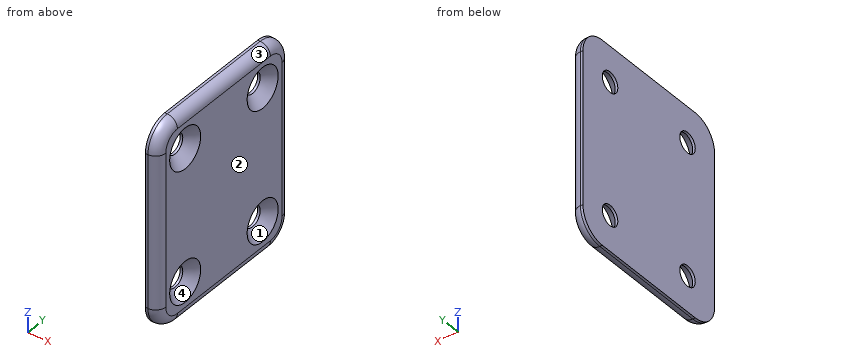
from build123d import *

# Parameters (mm, degrees)
CYLINDER005_R     = 2
CYLINDER005_DEPTH = 30
CYLINDER006_R     = 2
CYLINDER006_DEPTH = 30
CYLINDER007_R     = 2
CYLINDER007_DEPTH = 30
CYLINDER004_R     = 2
CYLINDER004_DEPTH = 30
BOX001_W          = 2.5
BOX001_H          = 34
BOX001_DEPTH      = 40
FILLET006_R       = 5
CHAMFER006_SIZE   = 2
FILLET007_R       = 2


with BuildPart() as obj1:
    # Cylinder005 → Cylinder005 (new body)
    with BuildSketch(Plane(origin=(20, -10, 6), x_dir=(0, 0, -1), z_dir=(1, 0, 0))):
        Circle(CYLINDER005_R)
    extrude(amount=CYLINDER005_DEPTH)


with BuildPart() as obj2:
    # Cylinder006 → Cylinder006 (new body)
    with BuildSketch(Plane(origin=(20, -10, 32), x_dir=(0, 0, -1), z_dir=(1, 0, 0))):
        Circle(CYLINDER006_R)
    extrude(amount=CYLINDER006_DEPTH)


with BuildPart() as obj3:
    # Cylinder007 → Cylinder007 (new body)
    with BuildSketch(Plane(origin=(20, 10, 6), x_dir=(0, 0, -1), z_dir=(1, 0, 0))):
        Circle(CYLINDER007_R)
    extrude(amount=CYLINDER007_DEPTH)


with BuildPart() as obj4:
    # Cylinder004 → Cylinder004 (new body)
    with BuildSketch(Plane(origin=(20, 10, 32), x_dir=(0, 0, -1), z_dir=(1, 0, 0))):
        Circle(CYLINDER004_R)
    extrude(amount=CYLINDER004_DEPTH)

    # Fusion003: union obj1, obj2, obj3
    add(obj1.part)
    add(obj2.part)
    add(obj3.part)


with BuildPart() as obj5:
    # Box001 → Box001 (new body)
    with BuildSketch(Plane(origin=(38, -17, -1), x_dir=(1, 0, 0), z_dir=(0, 0, 1))):
        with Locations((1.25, 17)):
            Rectangle(BOX001_W, BOX001_H)
    extrude(amount=BOX001_DEPTH)

    # Fillet006
    fillet006_edges = [obj5.edges().sort_by_distance(p)[0] for p in [
        (39.25, -17, -1),
        (39.25, -17, 39),
        (39.25, 17, -1),
        (39.25, 17, 39),
    ]]
    fillet(fillet006_edges, radius=FILLET006_R)

    # Cut003: cut obj4
    add(obj4.part, mode=Mode.SUBTRACT)

    # Chamfer006
    chamfer006_edges = [obj5.edges().sort_by_distance(p)[0] for p in [
        (40.5, 10, 8),
        (40.5, 10, 34),
        (40.5, -10, 8),
        (40.5, -10, 34),
    ]]
    chamfer(chamfer006_edges, length=CHAMFER006_SIZE)

    # Fillet007
    fillet007_edges = [obj5.edges().sort_by_distance(p)[0] for p in [
        (40.5, -17, 19),
    ]]
    fillet(fillet007_edges, radius=FILLET007_R)


solid = obj5.part
Geometry check sheet. Reference: the model listing, model coordinates, mm. Face numbers are marked on the shaded views. Give positions to 0.01 mm unless a question says otherwise; leave off trailing zeros. Loops run counter-clockwise (first coordinate to the right, second up) from the corner with the lowest first, then second, coordinate; pieces in that order, holes last.
(1) Release check for a two-part mould opening along Z. For the marked faces 1, 2, 3 and 4 record: released by +Z, released by -Z, zero draft, split by the parting line, or undercut.
From the geometry:
face 1: undercut
face 2: zero draft
face 3: released by +Z
face 4: undercut
(2) Section check A-A on y = 10. Record the cut outline in (x, z).
From the geometry:
outline: (38, -1) - (38.5, -1) arc R2 ccw to (40.5, 1) - (40.5, 2) - (38.5, 4) - (38, 4) - close; (38, 8) - (38.5, 8) - (40.5, 10) - (40.5, 28) - (38.5, 30) - (38, 30) - close; (38, 34) - (38.5, 34) - (40.5, 36) - (40.5, 37) arc R2 ccw to (38.5, 39) - (38, 39) - close
(3) Depth check by flat-ended pin: pin 1 Ø3 at (y, z) = (12, 34.5) entering from +X. Enter the tip coordinate at first touch or a pass-through.
From the geometry:
pin 1: stops at x = 40.5
(4) Section check B-B on z = 32. Record the cut outline in (x, y), then the cut area to 3 significant figures.
From the geometry:
outline: (38, -17) - (38.5, -17) arc R2 ccw to (40.5, -15) - (40.5, -14) - (38.5, -12) - (38, -12) - close; (38, -8) - (38.5, -8) - (40.5, -6) - (40.5, 6) - (38.5, 8) - (38, 8) - close; (38, 12) - (38.5, 12) - (40.5, 14) - (40.5, 15) arc R2 ccw to (38.5, 17) - (38, 17) - close
area: 55.3 mm2
(5) Thickness scan on L1, parallel to Z at x = 38.25, y = 10; L2, parallel to Y at x = 38.3, z = 6; L3, parallel to Z at x = 38.8, y = 9. Record the ranges inside material, lowest first.
From the geometry:
L1: z = -1 to 4, 8 to 30, 34 to 39
L2: y = -17 to -12, -8 to 8, 12 to 17
L3: z = -0.98 to 3.93, 8.07 to 29.93, 34.07 to 38.98
(6) Section check C-C on z = 12.5. Record the cut outline in (x, y), then the cut area to 3 significant figures.
From the geometry:
outline: (38, -17) - (38.5, -17) arc R2 ccw to (40.5, -15) - (40.5, 15) arc R2 ccw to (38.5, 17) - (38, 17) - close
area: 83.3 mm2
